Design review of the part built by this model. Coordinates are the model's own, in mm. Face numbers are marked on the shaded views. A direction names the side the tool comes from. Give positions to 0.01 mm unless a question says otherwise; leave off trailing zeros. Write each loop counter-clockwise with the first axis right and the second up, starting at its lowest first coordinate (ties: lowest second). Pieces come first, ordered by that corner, then holes. Notation, with made-up numbers: (-17.75, 9) -> (0.25, 9) arc R20 cw to (0.25, 28) -> close; hole circle Ø4 at (-12, 47.5). An arc over 180 degrees is marked (long way). Write each question's results on one line, items separated by ' | '. Start each with the question number.
(1) For the marked faces 1 and 2, list the 3-axis set-ups (+Z, -Z, +X, -X, +Y, -Y) from which the entire face can be reached by the end or side of a thin tool; tool diameter is ignored.
(2) Take a section at B-B (x = 3). State the section outline as (y, z) points, plus the area to 3 significant figures.
(3) To check wall thickness, follow probe 1 along Z at (x, y) = (6.5, -0.1); probe 2 along Z at (x, y) = (7, -0.4); probe 3 along Y at (x, z) = (-10, 13). State the ranges of each line that lie inside material, in increasing order.
(4) Take a section at C-C (z = -2.5). State the section outline as (x, y) points.
(5) Take a section at A-A (z = 12). State the section outline as (x, y) points, plus the area to 3 significant figures.
(6) Take a section at D-D (y = -2). Count the separate pieces of the cut face and the enclosed holes in it, plus the area to 3 significant figures.
from build123d import *

# Parameters (mm, degrees)
BOSS_EXTRUDE1_DEPTH = 2.38125
SKETCH1_4_W         = 7.14375
SKETCH1_4_H         = 10.31875
BOSS_EXTRUDE2_DEPTH = 3.302
SKETCH1_5_R         = 1.5875
CUT_EXTRUDE1_DEPTH  = 24.247602802


with BuildPart() as part:
    # Sketch1 → Boss-Extrude1 (new body)
    with BuildSketch(Plane(origin=(0, 0, 0), x_dir=(1, 0, 0), z_dir=(0, 1, 0))):
        with BuildLine():
            Line((12.969875, -16.271875), (-12.969875, -16.271875))
            ThreePointArc((-12.969875, -16.271875), (-15.304741591, -15.304741591), (-16.271875, -12.969875))
            Line((-16.271875, -12.969875), (-16.271875, 12.969875))
            ThreePointArc((-16.271875, 12.969875), (-15.304741591, 15.304741591), (-12.969875, 16.271875))
            Line((-12.969875, 16.271875), (12.969875, 16.271875))
            ThreePointArc((12.969875, 16.271875), (15.304741591, 15.304741591), (16.271875, 12.969875))
            Line((16.271875, 12.969875), (16.271875, -12.969875))
            ThreePointArc((16.271875, -12.969875), (15.304741591, -15.304741591), (12.969875, -16.271875))
        make_face()
    extrude(amount=-BOSS_EXTRUDE1_DEPTH)

    # Sketch1_4 → Boss-Extrude2 (add)
    with BuildSketch(Plane(origin=(0, 0, 0), x_dir=(1, 0, 0), z_dir=(0, 1, 0))):
        Rectangle(SKETCH1_4_W, SKETCH1_4_H)
    extrude(amount=BOSS_EXTRUDE2_DEPTH)

    # Sketch1_5 → Cut-Extrude1 (cut, through all)
    with BuildSketch(Plane(origin=(0, 0, 0), x_dir=(1, 0, 0), z_dir=(0, 1, 0))):
        with Locations(Location((-12.065, 12.065, 0), (0, 0, 270))):
            Circle(SKETCH1_5_R)
        with Locations(Location((-7.540625, -7.540625, 0), (0, 0, 270))):
            Circle(SKETCH1_5_R)
        with Locations(Location((7.540625, -7.540625, 0), (0, 0, 270))):
            Circle(SKETCH1_5_R)
        with Locations(Location((12.065, -12.065, 0), (0, 0, 270))):
            Circle(SKETCH1_5_R)
        with Locations(Location((12.065, 12.065, 0), (0, 0, 270))):
            Circle(SKETCH1_5_R)
        with Locations(Location((-7.540625, 7.540625, 0), (0, 0, 270))):
            Circle(SKETCH1_5_R)
        with Locations(Location((-12.065, -12.065, 0), (0, 0, 270))):
            Circle(SKETCH1_5_R)
        with Locations(Location((7.540625, 7.540625, 0), (0, 0, 270))):
            Circle(SKETCH1_5_R)
    extrude(amount=-CUT_EXTRUDE1_DEPTH, mode=Mode.SUBTRACT)


solid = part.part
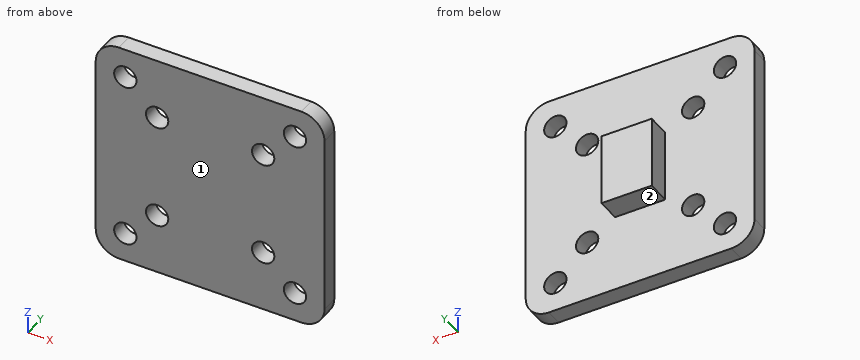
Report:
1) face 1: +Z, -Z, +X, -X, -Y | face 2: -Z, +X, -X, +Y
2) outline: (-2.38, -16.27) -> (0, -16.27) -> (0, -5.16) -> (3.3, -5.16) -> (3.3, 5.16) -> (0, 5.16) -> (0, 16.27) -> (-2.38, 16.27) -> close | area: 112 mm2
3) probe 1: -16.27 to -8.74, -6.34 to 6.34, 8.74 to 16.27 | probe 2: -16.27 to -9.03, -6.05 to 6.05, 9.03 to 16.27 | probe 3: -2.38 to 0
4) outline: (-16.27, -2.38) -> (16.27, -2.38) -> (16.27, 0) -> (3.57, 0) -> (3.57, 3.3) -> (-3.57, 3.3) -> (-3.57, 0) -> (-16.27, 0) -> close
5) outline: (-16.27, -2.38) -> (-13.65, -2.38) -> (-13.65, 0) -> (-16.27, 0) -> close; (-10.48, -2.38) -> (10.48, -2.38) -> (10.48, 0) -> (-10.48, 0) -> close; (13.65, -2.38) -> (16.27, -2.38) -> (16.27, 0) -> (13.65, 0) -> close | area: 62.4 mm2
6) separate pieces: 1 | enclosed holes: 8 | area: 986 mm2
